Verification items for the finished model (mm, model axes). Face numbers are marked on the shaded views. A direction names the side the tool comes from. Coordinates: 2 decimals unless noted, no trailing zeros. Write each loop counter-clockwise with the first axis right and the second up, starting at its lowest first coordinate (ties: lowest second). Pieces come first, ordered by that corner, then holes. Notation, with made-up numbers: M -14.5,-22 L 21.5,-22 A27 ccw 21.5,9 Z; hole C -15.5,56 d11. An arc over 180 degrees is marked long. Answer in a Markdown table with one row per item.
from build123d import *

# Parameters (mm, degrees)
SCHIZZO1_R                           = 5
BASE_FLANGIA1_DEPTH                  = 1.5
BORDO_FLANGIA1_STRIP_W               = 12
BORDO_FLANGIA1_STRIP_H               = 1.5
BORDO_FLANGIA1_STRIP_CUT_DEPTH       = 100
BORDO_FLANGIA1_STRIP_2_W             = 12
BORDO_FLANGIA1_STRIP_2_H             = 1.5
BORDO_FLANGIA1_STRIP_CUT_2_DEPTH     = 100
BORDO_FLANGIA1_DEPTH                 = 100
BORDO_FLANGIA1_BEND_DEPTH            = 100
BORDO_FLANGIA2_STRIP_W               = 7.4732
BORDO_FLANGIA2_STRIP_H               = 1.5
BORDO_FLANGIA2_STRIP_CUT_DEPTH       = 100
BORDO_FLANGIA2_STRIP_2_W             = 7.4732
BORDO_FLANGIA2_STRIP_2_H             = 1.5
BORDO_FLANGIA2_STRIP_CUT_2_DEPTH     = 100
BORDO_FLANGIA2_DEPTH                 = 100
BORDO_FLANGIA2_BEND_DEPTH            = 100
PIEGATURA_START                      = 58.9178
PIEGATURA_DELLO_SCHIZZO1_OUTLINE_W   = 20
PIEGATURA_DELLO_SCHIZZO1_OUTLINE_H   = 1.5
PIEGATURA_DELLO_SCHIZZO1_DEPTH       = 32.0822
PIEGATURA_START_2                    = 56.266894772
PIEGATURA_DELLO_SCHIZZO1_2_OUTLINE_R = 5
PIEGATURA_DELLO_SCHIZZO1_2_DEPTH     = 3.233105228
PIEGATURA_START_3                    = -10
PIEGATURA_DELLO_SCHIZZO1_3_DEPTH     = 20
PIEGATURA_DELLO_SCHIZZO1_4_DEPTH     = 20
SCHIZZO19_R                          = 6
TAGLIO_ESTRUSIONE1_DEPTH             = 138.567372501


with BuildPart() as part:
    # Base-Flangia1: sheet metal written as solids
    # Schizzo1 → Base-Flangia1 (new body)
    with BuildSketch(Plane(origin=(0, 0, 0), x_dir=(1, 0, 0), z_dir=(0, 1, 0))):
        with BuildLine():
            Line((10, 50), (10, 80))
            ThreePointArc((10, 80), (0, 90), (-10, 80))
            Line((-10, 80), (-10, 50))
            Line((-10, 50), (-50, 50))
            Line((-50, 50), (-50, -50))
            Line((-50, -50), (-10, -50))
            Line((-10, -50), (-10, -80))
            ThreePointArc((-10, -80), (0, -90), (10, -80))
            Line((10, -80), (10, -50))
            Line((10, -50), (50, -50))
            Line((50, -50), (50, 50))
            Line((50, 50), (10, 50))
        make_face()
        with Locations(Location((0, 80, 0), (0, 0, 270))):
            Circle(SCHIZZO1_R, mode=Mode.SUBTRACT)
        with Locations(Location((0, -80, 0), (0, 0, 270))):
            Circle(SCHIZZO1_R, mode=Mode.SUBTRACT)
    extrude(amount=-BASE_FLANGIA1_DEPTH)

    # Bordo-Flangia1: sheet metal written as solids
    # Bordo-Flangia1 strip (on a plane across the edge) → Bordo-Flangia1 strip cut (cut)
    with BuildSketch(Plane(origin=(-50, 0, -50), x_dir=(1, 0, 0), z_dir=(0, 0, 1))):
        with Locations((-1.5, -0.75)):
            Rectangle(BORDO_FLANGIA1_STRIP_W, BORDO_FLANGIA1_STRIP_H)
    extrude(amount=BORDO_FLANGIA1_STRIP_CUT_DEPTH, mode=Mode.SUBTRACT)

    # Bordo-Flangia1 strip 2 (on a plane across the edge) → Bordo-Flangia1 strip cut 2 (cut)
    with BuildSketch(Plane(origin=(50, 0, 50), x_dir=(-1, 0, 0), z_dir=(0, 0, -1))):
        with Locations((-1.5, -0.75)):
            Rectangle(BORDO_FLANGIA1_STRIP_2_W, BORDO_FLANGIA1_STRIP_2_H)
    extrude(amount=BORDO_FLANGIA1_STRIP_CUT_2_DEPTH, mode=Mode.SUBTRACT)

    # Bordo-Flangia1 section (on a plane across the edge) → Bordo-Flangia1 (add)
    with BuildSketch(Plane(origin=(-50, 0, -50), x_dir=(1, 0, 0), z_dir=(0, 0, 1))):
        with BuildLine():
            Line((0, 3), (0, 38.5))
            Line((0, 38.5), (1.5, 38.5))
            Line((1.5, 38.5), (1.5, 3))
            ThreePointArc((1.5, 3), (2.378679656, 0.878679656), (4.5, 0))
            Line((4.5, 0), (4.5, -1.5))
            ThreePointArc((4.5, -1.5), (1.318019485, -0.181980515), (0, 3))
        make_face()
    extrude(amount=BORDO_FLANGIA1_DEPTH)

    # Bordo-Flangia1 section 2 (on a plane across the edge) → Bordo-Flangia1 bend (add)
    with BuildSketch(Plane(origin=(50, 0, 50), x_dir=(-1, 0, 0), z_dir=(0, 0, -1))):
        with BuildLine():
            Line((0, 3), (0, 38.5))
            Line((0, 38.5), (1.5, 38.5))
            Line((1.5, 38.5), (1.5, 3))
            ThreePointArc((1.5, 3), (2.378679656, 0.878679656), (4.5, 0))
            Line((4.5, 0), (4.5, -1.5))
            ThreePointArc((4.5, -1.5), (1.318019485, -0.181980515), (0, 3))
        make_face()
    extrude(amount=BORDO_FLANGIA1_BEND_DEPTH)

    # Bordo-Flangia2: sheet metal written as solids
    # Bordo-Flangia2 strip (on a plane across the edge) → Bordo-Flangia2 strip cut (cut)
    with BuildSketch(Plane(origin=(50, 38.5, -50), x_dir=(0, -1, 0), z_dir=(0, 0, 1))):
        with Locations((-1.5, -0.75)):
            Rectangle(BORDO_FLANGIA2_STRIP_W, BORDO_FLANGIA2_STRIP_H)
    extrude(amount=BORDO_FLANGIA2_STRIP_CUT_DEPTH, mode=Mode.SUBTRACT)

    # Bordo-Flangia2 strip 2 (on a plane across the edge) → Bordo-Flangia2 strip cut 2 (cut)
    with BuildSketch(Plane(origin=(-50, 38.5, 50), x_dir=(0, -1, 0), z_dir=(0, 0, -1))):
        with Locations((-1.5, -0.75)):
            Rectangle(BORDO_FLANGIA2_STRIP_2_W, BORDO_FLANGIA2_STRIP_2_H)
    extrude(amount=BORDO_FLANGIA2_STRIP_CUT_2_DEPTH, mode=Mode.SUBTRACT)

    # Bordo-Flangia2 section (on a plane across the edge) → Bordo-Flangia2 (add)
    with BuildSketch(Plane(origin=(50, 38.5, -50), x_dir=(0, -1, 0), z_dir=(0, 0, 1))):
        with BuildLine():
            Line((0, 0.7366), (0, 25))
            Line((0, 25), (1.5, 25))
            Line((1.5, 25), (1.5, 0.7366))
            ThreePointArc((1.5, 0.7366), (1.715745145, 0.215745145), (2.2366, 0))
            Line((2.2366, 0), (2.2366, -1.5))
            ThreePointArc((2.2366, -1.5), (0.655084973, -0.844915027), (0, 0.7366))
        make_face()
    extrude(amount=BORDO_FLANGIA2_DEPTH)

    # Bordo-Flangia2 section 2 (on a plane across the edge) → Bordo-Flangia2 bend (add)
    with BuildSketch(Plane(origin=(-50, 38.5, 50), x_dir=(0, -1, 0), z_dir=(0, 0, -1))):
        with BuildLine():
            Line((0, 0.7366), (0, 25))
            Line((0, 25), (1.5, 25))
            Line((1.5, 25), (1.5, 0.7366))
            ThreePointArc((1.5, 0.7366), (1.715745145, 0.215745145), (2.2366, 0))
            Line((2.2366, 0), (2.2366, -1.5))
            ThreePointArc((2.2366, -1.5), (0.655084973, -0.844915027), (0, 0.7366))
        make_face()
    extrude(amount=BORDO_FLANGIA2_BEND_DEPTH)

    # Piegatura dello schizzo1: read off the stored shape, not the designer's step
    # Piegatura dello schizzo1 outline → Piegatura dello schizzo1 (cut)
    with BuildSketch(Plane.XY.offset(PIEGATURA_START)):
        with Locations((0, -0.75)):
            Rectangle(PIEGATURA_DELLO_SCHIZZO1_OUTLINE_W, PIEGATURA_DELLO_SCHIZZO1_OUTLINE_H)
    extrude(amount=PIEGATURA_DELLO_SCHIZZO1_DEPTH, mode=Mode.SUBTRACT)

    # Piegatura dello schizzo1 2 outline → Piegatura dello schizzo1 2 (add)
    with BuildSketch(Plane.XY.offset(PIEGATURA_START_2)):
        with BuildLine():
            Line((10, -23.609513775), (10, -1.5))
            Line((10, -1.5), (-10, -1.5))
            Line((-10, -1.5), (-10, -23.609513775))
            ThreePointArc((-10, -23.609513775), (0, -33.609513775), (10, -23.609513775))
        make_face()
        with Locations((0, -23.609513775)):
            Circle(PIEGATURA_DELLO_SCHIZZO1_2_OUTLINE_R, mode=Mode.SUBTRACT)
    extrude(amount=PIEGATURA_DELLO_SCHIZZO1_2_DEPTH)

    # Piegatura dello schizzo1 3 outline → Piegatura dello schizzo1 3 (cut)
    with BuildSketch(Plane.YZ.offset(PIEGATURA_START_3)):
        with BuildLine():
            ThreePointArc((-1.780629183, 56.266894772), (-2.887654552, 57.529889753), (-4.5, 58))
            Line((-4.5, 58), (-35, 58))
            Line((-35, 58), (-35, 56.266894772))
            Line((-35, 56.266894772), (-1.780629183, 56.266894772))
        make_face()
        with BuildLine():
            Line((1, 54), (1, 58.9178))
            Line((1, 58.9178), (-1.5, 58.9178))
            Line((-1.5, 58.9178), (-1.5, 61))
            Line((-1.5, 61), (-35, 61))
            Line((-35, 61), (-35, 59.500000008))
            Line((-35, 59.500000008), (-4.5, 59.5))
            ThreePointArc((-4.5, 59.5), (-1.318019485, 58.181980515), (0, 55))
            Line((0, 55), (0, 54))
            Line((0, 54), (1, 54))
        make_face()
    extrude(amount=PIEGATURA_DELLO_SCHIZZO1_3_DEPTH, mode=Mode.SUBTRACT)

    # Piegatura dello schizzo1 4 outline → Piegatura dello schizzo1 4 (add)
    with BuildSketch(Plane.YZ.offset(PIEGATURA_START_3)):
        with BuildLine():
            Line((-0.182016948, 56.266894772), (-1.780629183, 56.266894772))
            ThreePointArc((-1.780629183, 56.266894772), (-1.570997401, 55.6488018), (-1.5, 55))
            Line((-1.5, 55), (-1.500000001, 54))
            Line((-1.500000001, 54), (0, 54))
            Line((0, 54), (0, 55))
            ThreePointArc((0, 55), (-0.045736664, 55.639951665), (-0.182016948, 56.266894772))
        make_face()
    extrude(amount=PIEGATURA_DELLO_SCHIZZO1_4_DEPTH)

    # Schizzo19 → Taglio-Estrusione1 (cut, through all)
    with BuildSketch(Plane(origin=(0, 38.5, 0), x_dir=(1, 0, 0), z_dir=(0, 1, 0))):
        with Locations(Location((-60, 35, 0), (0, 0, 270))):
            Circle(SCHIZZO19_R)
        with Locations(Location((-60, -35, 0), (0, 0, 90))):
            Circle(SCHIZZO19_R)
        with Locations(Location((60, -35, 0), (0, 0, 270))):
            Circle(SCHIZZO19_R)
        with Locations(Location((60, 35, 0), (0, 0, 90))):
            Circle(SCHIZZO19_R)
    extrude(amount=-TAGLIO_ESTRUSIONE1_DEPTH, mode=Mode.SUBTRACT)


solid = part.part
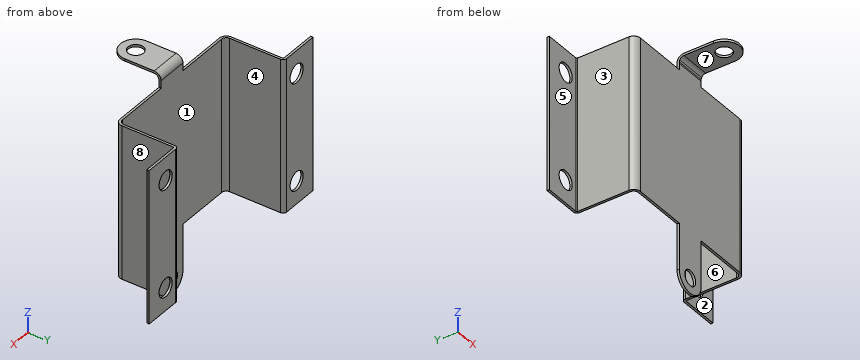
1) Sectioned sample at A-A (x = -60). Record the cut outline in (y, z), then the cut area to 3 significant figures.
Response values:
| item | result |
|---|---|
| outline | M 37,-50 L 38.5,-50 L 38.5,-41 L 37,-41 Z; M 37,-29 L 38.5,-29 L 38.5,29 L 37,29 Z; M 37,41 L 38.5,41 L 38.5,50 L 37,50 Z |
| area | 114 mm² |
2) Thickness scan on L1, parallel to X at y = 2.5, z = 2; L2, parallel to X at y = 38.1, z = 35; L3, parallel to Y at x = 67.5, z = 3. Record the ranges inside material, lowest first. Write a range as [from, to].
Response values:
| item | result |
|---|---|
| L1 | x = [-49.97, -48.46], [48.46, 49.97] |
| L2 | x = [-75, -66], [-54, -49.46], [49.46, 54], [66, 75] |
| L3 | y = [37, 38.5] |
3) Sectioned sample at B-B (z = 35). Record the cut outline in (x, y).
Response values:
| item | result |
|---|---|
| outline | M -75,37 L -66,37 L -66,38.5 L -75,38.5 Z; M -54,37 L -50.74,37 A0.74 cw -50,36.26 L -50,3 A4.5 ccw -45.5,-1.5 L 45.5,-1.5 A4.5 ccw 50,3 L 50,36.26 A0.74 cw 50.74,37 L 54,37 L 54,38.5 L 50.74,38.5 A2.24 ccw 48.5,36.26 L 48.5,3 A3 cw 45.5,0 L -45.5,0 A3 cw -48.5,3 L -48.5,36.26 A2.24 ccw -50.74,38.5 L -54,38.5 Z; M 66,37 L 75,37 L 75,38.5 L 66,38.5 Z |
4) Sectioned sample at C-C (y = 16). Record the cut outline in (x, z).
Response values:
| item | result |
|---|---|
| outline | M -50,-50 L -48.5,-50 L -48.5,50 L -50,50 Z; M 48.5,-50 L 50,-50 L 50,50 L 48.5,50 Z |
5) Release check for a two-part mould opening along X. For the marked faces 1, 2, 3 and 4 record: +X half, -X half, draft (parallel to the pull), parting line (faces both ways), or undercut.
Response values:
| item | result |
|---|---|
| face 1 | undercut |
| face 2 | draft |
| face 3 | -X half |
| face 4 | undercut |
6) Sectioned sample at D-D (z = 9.5). Record the cut outline in (x, y), then the cut area to 3 significant figures.
Response values:
| item | result |
|---|---|
| outline | M -75,37 L -50.74,37 A0.74 cw -50,36.26 L -50,3 A4.5 ccw -45.5,-1.5 L 45.5,-1.5 A4.5 ccw 50,3 L 50,36.26 A0.74 cw 50.74,37 L 75,37 L 75,38.5 L 50.74,38.5 A2.24 ccw 48.5,36.26 L 48.5,3 A3 cw 45.5,0 L -45.5,0 A3 cw -48.5,3 L -48.5,36.26 A2.24 ccw -50.74,38.5 L -75,38.5 Z |
| area | 334 mm² |
7) Tool access check on the marked faces 5, 6, 7 and 8. Record the directions out of +Z, -Z, +X, -X, +Y, -Y that give a thin tool (end or side, any length) a straight path to the whole face; none if there is none.
Response values:
| item | result |
|---|---|
| face 5 | +Z, -Z, -X, -Y |
| face 6 | +Z, -Z, +Y |
| face 7 | -Z, +X, -X, -Y |
| face 8 | +Z, -Z, +X, -Y |
8) Depth check by flat-ended pin: pin 1 (13 mm diameter, centred on x = 0, y = -23.61, fed in from -Z); pin 2 (12 mm diameter, centred on x = -62.5, z = 21, fed in from -Y); pin 3 (5 mm diameter, centred on x = 13, z = -42.5, fed in from +Y); pin 4 (11 mm diameter, centred on x = 60, z = -35, fed in from +Y). Enter the tip coordinate at first touch or a pass-through.
Response values:
| item | result |
|---|---|
| pin 1 | stops at z = 58 |
| pin 2 | stops at y = 37 |
| pin 3 | stops at y = 0 |
| pin 4 | passes through |
